Design review of the part built by this model. Coordinates are the model's own, in mm. Face numbers are marked on the shaded views. A direction names the side the tool comes from. Coordinates: 2 decimals unless noted, no trailing zeros. Loops run counter-clockwise (first coordinate to the right, second up) from the corner with the lowest first, then second, coordinate; pieces in that order, holes last.
Q1. Add section C-C on x = -12.7. Give the boundary of the cut face in (y, z), and give its area (3 significant figures).
Q2. Wall thickness on probe 1 along X at (y, z) = (-4.25, 1.25); probe 2 along Z at (x, y) = (12.7, -5.8); probe 3 along X at (y, z) = (-1.25, 2): over which ranges is each line inside the solid? List them lowest first.
Q3. Add section B-B on z = -2. Give the boundary of the cut face in (x, y) (3 decimals), and give its area (3 significant figures).
Q4. For P1, Ø1, axis at y = 0, z = 0.5, coming from the +X side; P2, Ø3, axis at y = 9.5, z = -2, coming from the +X side; P3, Ø2.5, axis at x = -12.7, z = 0, coming from the -Y side; P4, Ø3, axis at x = 4.5, y = 0, coming from the +Z side, all flat-tipped, find the tip position at first contact; note any pin that passes through.
Q5. Machinability: for the marked faces 1, 2 and 3, which of the approach directions +Z, -Z, +X, -X, +Y, -Y give a long, thin tool a straight path to every point of the face, cutting with its end or side? Answer none if there is none.
Q6. Add section A-A on y = -5.25. Give the boundary of the cut face in (x, z), and give its area (3 significant figures).
Q7. Add section D-D on z = -0.5. Give the boundary of the cut face in (x, y) (3 decimals).
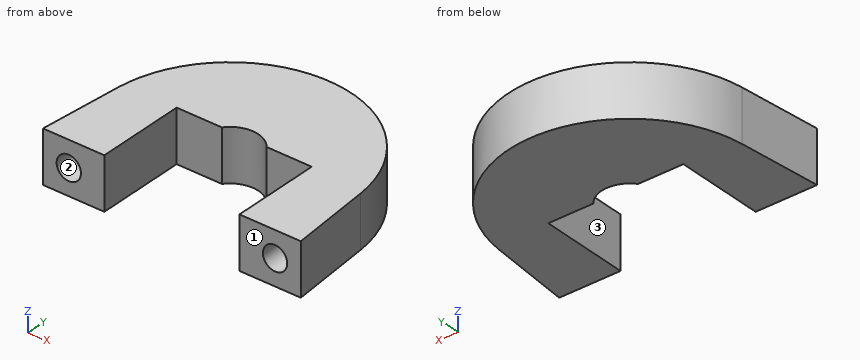
```python
from build123d import *

# Parameters (mm, degrees)
SALIENTE_EXTRUIR1_DEPTH = 3.2
CROQUIS2_R              = 1.5
CORTAR_EXTRUIR1_DEPTH   = 5


with BuildPart() as part:
    # Croquis1 → Saliente-Extruir1 (new, symmetric)
    with BuildSketch(Plane.XY):
        with BuildLine():
            Line((15.875, -8.77), (8.32, -8.77))
            Line((8.32, -8.77), (8.32, 2.157309855))
            Line((8.32, 2.157309855), (2.756086753, 2.157309855))
            ThreePointArc((2.756086753, 2.157309855), (0, 3.5), (-2.756086753, 2.157309855))
            Line((-2.756086753, 2.157309855), (-8.32, 2.157309855))
            Line((-8.32, 2.157309855), (-8.32, -8.77))
            Line((-8.32, -8.77), (-15.875, -8.77))
            Line((-15.875, -8.77), (-14.93627212, 1.381222339))
            ThreePointArc((-14.93627212, 1.381222339), (0, 15), (14.93627212, 1.381222339))
            Line((14.93627212, 1.381222339), (15.875, -8.77))
        make_face()
    extrude(amount=SALIENTE_EXTRUIR1_DEPTH, both=True)

    # Croquis2 → Cortar-Extruir1 (cut)
    with BuildSketch(Plane.XZ.offset(8.77)):
        with Locations((-12.7, 0)):
            Circle(CROQUIS2_R)
        with Locations(Location((12.7, 0, 0), (0, 0, 180))):
            Circle(CROQUIS2_R)
    extrude(amount=-CORTAR_EXTRUIR1_DEPTH, mode=Mode.SUBTRACT)


solid = part.part
```
Entries:
1. outline: (-8.77, -3.2) - (7.98, -3.2) - (7.98, 3.2) - (-8.77, 3.2) - (-8.77, 1.5) - (-3.77, 1.5) - (-3.77, -1.5) - (-8.77, -1.5) - close
1. area: 92.2 mm2
2. probe 1: x = -15.46 to -13.53, -11.87 to -8.32, 8.32 to 11.87, 13.53 to 15.46
2. probe 2: z = -3.2 to -1.5, 1.5 to 3.2
2. probe 3: x = -15.18 to -8.32, 8.32 to 15.18
3. outline: (-15.875, -8.77) - (-8.32, -8.77) - (-8.32, 2.157) - (-2.756, 2.157) arc R3.5 cw to (2.756, 2.157) - (8.32, 2.157) - (8.32, -8.77) - (15.875, -8.77) - (14.936, 1.381) arc R15 ccw to (-14.936, 1.381) - close
3. area: 438 mm2
4. P1: stops at x = 15.11
4. P2: stops at x = 12.69
4. P3: stops at y = -3.77
4. P4: passes through
5. face 1: +Z, -Z, +X, -X, -Y
5. face 2: -Y
5. face 3: +Z, -Z, -Y
6. outline: (-15.55, -3.2) - (-8.32, -3.2) - (-8.32, 3.2) - (-15.55, 3.2) - close; (8.32, -3.2) - (15.55, -3.2) - (15.55, 3.2) - (8.32, 3.2) - close; hole circle Ø3 at (-12.7, 0); hole circle Ø3 at (12.7, 0)
6. area: 78.4 mm2
7. outline: (-15.875, -8.77) - (-14.114, -8.77) - (-14.114, -3.77) - (-11.286, -3.77) - (-11.286, -8.77) - (-8.32, -8.77) - (-8.32, 2.157) - (-2.756, 2.157) arc R3.5 cw to (2.756, 2.157) - (8.32, 2.157) - (8.32, -8.77) - (11.286, -8.77) - (11.286, -3.77) - (14.114, -3.77) - (14.114, -8.77) - (15.875, -8.77) - (14.936, 1.381) arc R15 ccw to (-14.936, 1.381) - close
